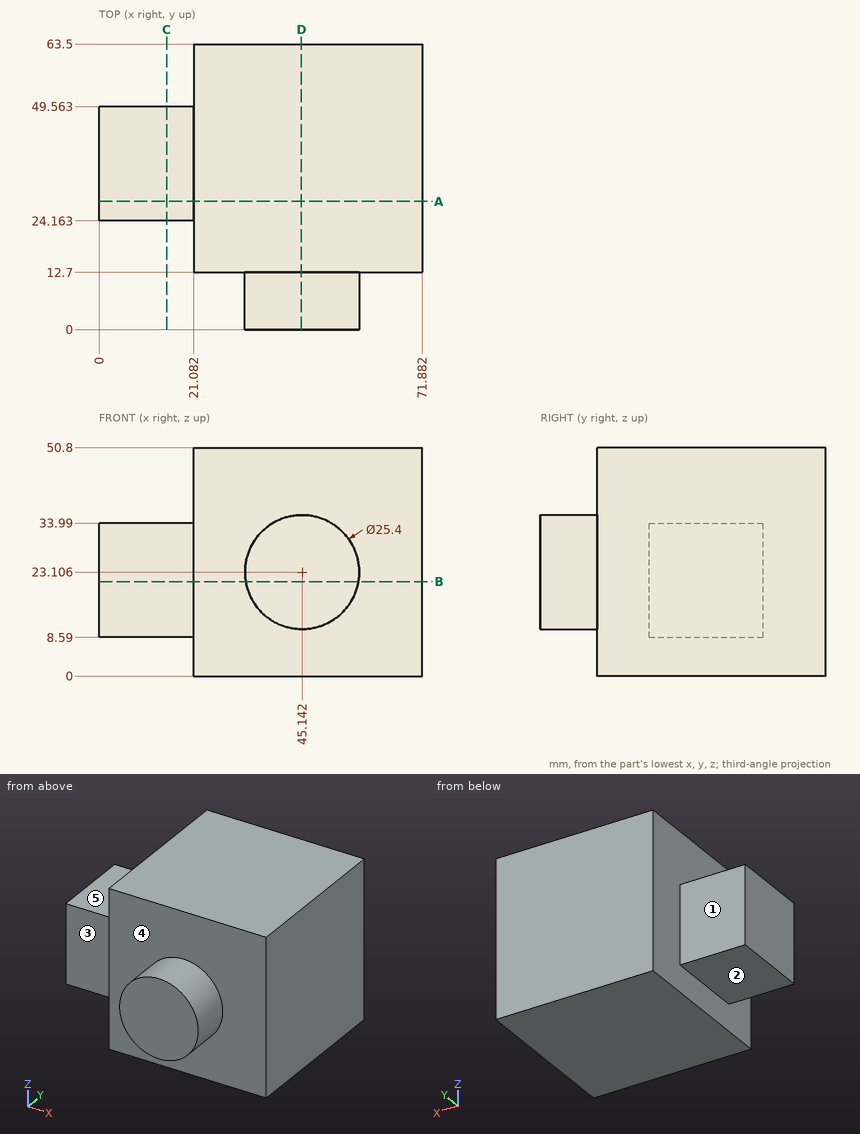
The drawing under review shows one solid part. Ordinate dimensions are in mm from its lowest x, y, z. A direction names the side the tool comes from. Round coordinates to 2 decimals unless told otherwise and drop trailing zeros. Write each loop counter-clockwise with the first axis right and the second up, starting at its lowest first coordinate (ties: lowest second). Pieces come first, ordered by that corner, then holes. Notation, with made-up numbers: (43, 61.5) -> (85, 61.5) arc R32 ccw to (85, 89.5) -> close; hole circle Ø9 at (81.25, 24.5). An arc over 180 degrees is marked (long way). One line per question, with ' | ' between items. Start each with the question number.
(1) Add section B-B, the plane z = 21. Write out the cut boundary in (x, y), plus the area to 3 significant figures.
(2) For line 1 along Z through (x, y) = (6, 44.5); line 2 along X through (y, z) = (33, 7.5); line 3 along Y through (x, z) = (64.5, 19), list the stretches that pass through material, from the lowest coordinate up. Write a range as from..to.
(3) Add section A-A, the plane y = 28.5. Write out the cut boundary in (x, z), plus the area to 3 significant figures.
(4) Insertion check: P1, Ø17, axis at x = 5.5, z = 15.5, coming from the +Y side; P2, Ø1.5, axis at y = 18, z = 44.5, coming from the -X side; P3, Ø23, axis at x = 14.5, z = 24.5, coming from the -Y side. Each pin has a flat end and moves straight along its axis. Give the tip position at first contact, or say it passes through.
(5) Add section C-C, the plane x = 15. Write out the cut boundary in (y, z).
(6) Add section D-D, the plane x = 45. Write out the cut boundary in (y, z) (1 decimal).
(7) Tool access review of the marked faces 1, 2, 3, 4 and 5: name each direction out of +Z, -Z, +X, -X, +Y, -Y from which nothing blocks a thin tool from reaching the whole face with its end or side.
Answer list:
1) outline: (0, 24.16) -> (21.08, 24.16) -> (21.08, 12.7) -> (32.62, 12.7) -> (32.62, 0) -> (57.67, 0) -> (57.67, 12.7) -> (71.88, 12.7) -> (71.88, 63.5) -> (21.08, 63.5) -> (21.08, 49.56) -> (0, 49.56) -> close | area: 3,430 mm²
2) line 1: 8.59..33.99 | line 2: 21.08..71.88 | line 3: 12.7..63.5
3) outline: (0, 8.59) -> (21.08, 8.59) -> (21.08, 0) -> (71.88, 0) -> (71.88, 50.8) -> (21.08, 50.8) -> (21.08, 33.99) -> (0, 33.99) -> close | area: 3,120 mm²
4) P1: y = 49.56 | P2: x = 21.08 | P3: y = 12.7
5) outline: (24.16, 8.59) -> (49.56, 8.59) -> (49.56, 33.99) -> (24.16, 33.99) -> close
6) outline: (0, 10.4) -> (12.7, 10.4) -> (12.7, 0) -> (63.5, 0) -> (63.5, 50.8) -> (12.7, 50.8) -> (12.7, 35.8) -> (0, 35.8) -> close
7) face 1: +Z, -Z, -X, +Y | face 2: -Z, -X, +Y, -Y | face 3: +Z, -Z, -X, -Y | face 4: -Y | face 5: +Z, -X, +Y, -Y
